Verification items for the finished model (mm, model axes). A direction names the side the tool comes from. Give positions to 0.01 mm unless a question says otherwise; leave off trailing zeros. Write each loop counter-clockwise with the first axis right and the second up, starting at its lowest first coordinate (ties: lowest second). Pieces come first, ordered by that corner, then holes.
Solid Edge part; units mm, degrees
sketch "Sketch1" plane through (0, 0, 0) normal (0, 0, 1) x (1, 0, 0)
  line L0 (0, 34) -> (0, 26)
  line L1 (0, 26) -> (-6, 26)
  line L2 (-6, 26) -> (-18.8863, 13.1137)
  line L3 (-18.8863, 13.1137) -> (-18.8863, -13.1137)
  line L4 (-18.8863, -13.1137) -> (-6, -26)
  line L5 (-6, -26) -> (0, -26)
  line L6 (0, -26) -> (0, -34)
  line L7 (0, -34) -> (-6.4853, -34)
  line L8 (-6.4853, -34) -> (-25, -15.4853)
  line L9 (-25, -15.4853) -> (-25, 15.4853)
  line L10 (-25, 15.4853) -> (-6.4853, 34)
  line L11 (-6.4853, 34) -> (0, 34)
extrude "Protrusion1" add sketch "Sketch1" along normal mid plane 6
sketch "Sketch2" plane through (0, 0, 0) normal (0, 0, 1) x (1, 0, 0)
  line L0 (-6, -26) -> (0, -26)
  line L1 (0, -26) -> (0, -41)
  line L2 (0, -41) -> (-6, -41)
  line L3 (-6, -41) -> (-6, -26)
extrude "ExtrudedProtrusion_2" add sketch "Sketch2" along normal mid plane 6
sketch "Sketch3" plane through (-12.2288, -3.5, -3) normal (0, 0, -1) x (0, 1, 0)
  line L0 (16.6137, -6.6575) -> (16.6137, -12.7712)
  line L1 (16.6137, -12.7712) -> (18.9853, -12.7712)
  line L2 (18.9853, -12.7712) -> (37.5, 5.7435)
  line L3 (37.5, 5.7435) -> (37.5, 12.2288)
  line L4 (37.5, 12.2288) -> (29.5, 12.2288)
  line L5 (29.5, 12.2288) -> (29.5, 6.2288)
  line L6 (29.5, 6.2288) -> (16.6137, -6.6575)
extrude "Cutout1" cut sketch "Sketch3" against normal through all
sketch "Sketch4" plane through (0, 0, 0) normal (0, 0, 1) x (1, 0, 0)
  line L0 (-18.8863, 13.1137) -> (-25, 13.1137)
  line L1 (-25, 13.1137) -> (-25, 28.1137)
  line L2 (-25, 28.1137) -> (-15, 38.1137)
  line L3 (-15, 38.1137) -> (-15, 43.1137)
  line L4 (-15, 43.1137) -> (-10, 43.1137)
  line L5 (-10, 43.1137) -> (-10, 23.1137)
  line L6 (-10, 23.1137) -> (-18.8863, 23.1137)
  line L7 (-18.8863, 23.1137) -> (-18.8863, 13.1137)
  dimension "D1" = 18.8863
  dimension "D2" = 25
  dimension "D3" = 15
extrude "ExtrudedProtrusion_3" add sketch "Sketch4" along normal mid plane 6
hole "Hole_1" at (-16, 29.1137, -3) direction (0, 0, 1) diameter 5 end up to next
properties material "Polyethylene, low density"
Item 1: Scan lines: line 1 along Y through (x, z) = (-16.75, 0.4); line 2 along Y through (x, z) = (-16, -1.4); line 3 along X through (y, z) = (10.5, 0.9). Record each from-to range of solid material in increasing order.
Answer key:
line 1: y = -23.74 to -15.25, 23.11 to 26.73, 31.5 to 36.36
line 2: y = -24.49 to -16, 23.11 to 26.61, 31.61 to 37.11
line 3: x = -25 to -18.89
Item 2: Sectioned sample at B-B on x = -16. Record the cut outline in (y, z), then the cut area to 3 significant figures.
Answer key:
outline: (-24.49, -3) - (-16, -3) - (-16, 3) - (-24.49, 3) - close; (23.11, -3) - (26.61, -3) - (26.61, 3) - (23.11, 3) - close; (31.61, -3) - (37.11, -3) - (37.11, 3) - (31.61, 3) - close
area: 105 mm2
Item 3: Set-up check for faces 1 (the face through (-13, -19, 0)), 2 (the face through (-15, 41, 0)), 3 (the face through (-6, -38, 0)), 4 (the face through (-3, -26, 0)): record each of +Z, -Z, +X, -X, +Y, -Y from which the full face is reachable in a straight line by a thin tool's end or side.
Answer key:
face 1: +Z, -Z, +X
face 2: +Z, -Z, -X, +Y
face 3: +Z, -Z, -X, -Y
face 4: +Z, -Z, +X, +Y
Item 4: Sectioned sample at C-C on y = -5.5. Record the cut outline in (x, z).
Answer key:
outline: (-25, -3) - (-18.89, -3) - (-18.89, 3) - (-25, 3) - close
Item 5: Release check for a two-part mould opening along X. For faces 5 (the face through (-20.07, 33.044, -0.042)), 6 (the face through (-13, 43.114, 0)), 7 (the face through (0, -33, 0)), 8 (the face through (-18.44, 28.57, -0.04)) record: released by +X, released by -X, zero draft, split by the parting line, or undercut.
Answer key:
face 5: released by -X
face 6: zero draft
face 7: released by +X
face 8: undercut
Item 6: Depth check by flat-ended pin: pin 1 (1.8 mm diameter, centred on y = 31, z = -1.5, fed in from +X); pin 2 (3 mm diameter, centred on x = -16, y = 29.11, fed in from +Z); pin 3 (2.5 mm diameter, centred on y = 41.5, z = 0.5, fed in from -X); pin 4 (3 mm diameter, centred on y = -37, z = 1, fed in from -X). Enter the tip coordinate at first touch or a pass-through.
Answer key:
pin 1: stops at x = -10
pin 2: passes through
pin 3: stops at x = -15
pin 4: stops at x = -6
Item 7: Sectioned sample at D-D on x = -7.25. Record the cut outline in (y, z), then the cut area to 3 significant figures.
Answer key:
outline: (-33.24, -3) - (-24.75, -3) - (-24.75, 3) - (-33.24, 3) - close
area: 50.9 mm2
Item 8: Sectioned sample at A-A on z = 0.85. Record the cut outline in (x, y), then the cut area to 3 significant figures.
Answer key:
outline: (-25, -15.49) - (-6.49, -34) - (-6, -34) - (-6, -41) - (0, -41) - (0, -26) - (-6, -26) - (-18.89, -13.11) - (-18.89, 23.11) - (-10, 23.11) - (-10, 43.11) - (-15, 43.11) - (-15, 38.11) - (-25, 28.11) - close; hole circle Ø5 at (-16, 29.11)
area: 634 mm2
